from build123d import *

# Parameters (mm, degrees)
SKETCH1_W            = 85.09
SKETCH1_H            = 56.64
BOSS_EXTRUDE1_DEPTH  = 2
SKETCH3_W            = 6
SKETCH3_H            = 2
BOSS_EXTRUDE4_DEPTH  = 6
SKETCH4_R            = 1.27
CUT_EXTRUDE3_DEPTH   = 6
SKETCH5_W            = 6
SKETCH5_H            = 2
BOSS_EXTRUDE5_DEPTH  = 6
SKETCH7_R            = 1.27
CUT_EXTRUDE4_DEPTH   = 6
SKETCH8_W            = 6
SKETCH8_H            = 2
BOSS_EXTRUDE6_DEPTH  = 6
SKETCH9_W            = 6
SKETCH9_H            = 2
BOSS_EXTRUDE7_DEPTH  = 6
SKETCH10_R           = 1.27
CUT_EXTRUDE5_DEPTH   = 6
SKETCH11_R           = 1.27
CUT_EXTRUDE6_DEPTH   = 6
FILLET5_R            = 2
SKETCH12_W           = 33.5
SKETCH12_H           = 5.2
BOSS_EXTRUDE8_DEPTH  = 15
SKETCH14_W           = 33.4
SKETCH14_H           = 5
CUT_EXTRUDE9_DEPTH   = 6
SKETCH15_W           = 5
SKETCH15_H           = 33
BOSS_EXTRUDE9_DEPTH  = 9
SKETCH16_W           = 85
SKETCH16_H           = 55
BOSS_EXTRUDE10_DEPTH = 3.5


with BuildPart() as part:
    # Sketch1 → Boss-Extrude1 (new body)
    with BuildSketch(Plane(origin=(0, 0, 0), x_dir=(1, 0, 0), z_dir=(0, 1, 0))):
        Rectangle(SKETCH1_W, SKETCH1_H)
    extrude(amount=BOSS_EXTRUDE1_DEPTH)

    # Sketch3 → Boss-Extrude4 (add)
    with BuildSketch(Plane(origin=(42.545, 0, 0), x_dir=(0, 0, -1), z_dir=(1, 0, 0))):
        with Locations((-25.32, 1)):
            Rectangle(SKETCH3_W, SKETCH3_H)
    extrude(amount=BOSS_EXTRUDE4_DEPTH)

    # Sketch4 → Cut-Extrude3 (cut)
    with BuildSketch(Plane(origin=(0, 2, 0), x_dir=(1, 0, 0), z_dir=(0, 1, 0))):
        with Locations((45.545, -25.32)):
            Circle(SKETCH4_R)
    extrude(amount=-CUT_EXTRUDE3_DEPTH, mode=Mode.SUBTRACT)

    # Sketch5 → Boss-Extrude5 (add)
    with BuildSketch(Plane(origin=(42.545, 0, 0), x_dir=(0, 0, -1), z_dir=(1, 0, 0))):
        with Locations((25.32, 1)):
            Rectangle(SKETCH5_W, SKETCH5_H)
    extrude(amount=BOSS_EXTRUDE5_DEPTH)

    # Sketch7 → Cut-Extrude4 (cut)
    with BuildSketch(Plane(origin=(0, 2, 0), x_dir=(1, 0, 0), z_dir=(0, 1, 0))):
        with Locations((45.545, 25.32)):
            Circle(SKETCH7_R)
    extrude(amount=-CUT_EXTRUDE4_DEPTH, mode=Mode.SUBTRACT)

    # Sketch8 → Boss-Extrude6 (add)
    with BuildSketch(Plane.ZY.offset(42.545)):
        with Locations((-25.32, 1)):
            Rectangle(SKETCH8_W, SKETCH8_H)
    extrude(amount=BOSS_EXTRUDE6_DEPTH)

    # Sketch9 → Boss-Extrude7 (add)
    with BuildSketch(Plane.ZY.offset(42.545)):
        with Locations((25.32, 1)):
            Rectangle(SKETCH9_W, SKETCH9_H)
    extrude(amount=BOSS_EXTRUDE7_DEPTH)

    # Sketch10 → Cut-Extrude5 (cut)
    with BuildSketch(Plane(origin=(0, 2, 0), x_dir=(1, 0, 0), z_dir=(0, 1, 0))):
        with Locations((-45.545, 25.32)):
            Circle(SKETCH10_R)
    extrude(amount=-CUT_EXTRUDE5_DEPTH, mode=Mode.SUBTRACT)

    # Sketch11 → Cut-Extrude6 (cut)
    with BuildSketch(Plane(origin=(0, 2, 0), x_dir=(1, 0, 0), z_dir=(0, 1, 0))):
        with Locations((-45.545, -25.32)):
            Circle(SKETCH11_R)
    extrude(amount=-CUT_EXTRUDE6_DEPTH, mode=Mode.SUBTRACT)

    # Fillet5
    fillet5_edges = [part.edges().sort_by_distance(p)[0] for p in [
        (48.545, 1, 28.32),
        (48.545, 1, 22.32),
        (48.545, 1, -28.32),
        (48.545, 1, -22.32),
        (-48.545, 1, -28.32),
        (-48.545, 1, -22.32),
        (-48.545, 1, 28.32),
        (-48.545, 1, 22.32),
    ]]
    fillet(fillet5_edges, radius=FILLET5_R)

    # Sketch12 → Boss-Extrude8 (add)
    with BuildSketch(Plane.XZ):
        with Locations((-24.795, -24.72)):
            Rectangle(SKETCH12_W, SKETCH12_H)
    extrude(amount=BOSS_EXTRUDE8_DEPTH)

    # Sketch14 → Cut-Extrude9 (cut)
    with BuildSketch(Plane.XZ.offset(15)):
        with Locations((-24.845, -24.72)):
            Rectangle(SKETCH14_W, SKETCH14_H)
    extrude(amount=-CUT_EXTRUDE9_DEPTH, mode=Mode.SUBTRACT)

    # Sketch15 → Boss-Extrude9 (add)
    with BuildSketch(Plane.XZ):
        with Locations((-37.045, 0.82)):
            Rectangle(SKETCH15_W, SKETCH15_H)
    extrude(amount=BOSS_EXTRUDE9_DEPTH)

    # Sketch16 → Boss-Extrude10 (add)
    with BuildSketch(Plane(origin=(0, 2, 0), x_dir=(1, 0, 0), z_dir=(0, 1, 0))):
        Rectangle(SKETCH16_W, SKETCH16_H)
    extrude(amount=BOSS_EXTRUDE10_DEPTH)


solid = part.part
Input: part model. Units: mm. Frame: model coordinates. A direction names the side the tool comes from. Round coordinates to 2 decimals unless told otherwise and drop trailing zeros. Loops run counter-clockwise (first coordinate to the right, second up) from the corner with the lowest first, then second, coordinate; pieces in that order, holes last. Notation, with made-up numbers: (73, -23) -> (108, -23) arc R27 cw to (108, 3) -> close; hole circle Ø2 at (-24, 34.25). An arc over 180 degrees is marked (long way). Answer as a JSON object with one key per item and string values. Group by question number.
1) Section query D-D on z = -19.5. Output: boundary loops of the cut face in (x, y) (3 decimals).
2) Section query A-A on z = -25.32. Output: boundary loops of the cut face in (x, y) (3 decimals).
3) Section query C-C on y = -4.5. Output: boundary loops of the cut face in (x, z) (3 decimals), plus the area to 3 significant figures.
4) Ray query, L1, parallel to X at y = 1.4, z = 25.32 (3 decimals); L2, parallel to Z at x = -18, y = -4; L3, parallel to Y at x = -1.5, z = 18. Return the intervals inside material, ascending.
5) Reachability of faces 5 (the flat face through (-25, -7, -27.32)), 6 (the flat face through (-25, -9, -25)), 7 (the flat face through (42.545, 1, 0)), 8 (the flat face through (-45, 1, -22.32)), 9 (the cylindrical face through (-46.553, 1.014, 26.093)) from +Z, -Z, +X, -X, +Y, -Y: full face, straight path, thin tool, end or side. Return the list, or none.
6) Pin query (flat end, axial travel): pin 1 (1.5 mm diameter, centred on y = -12, z = -25, fed in from -X) (3 decimals); pin 2 (4 mm diameter, centred on y = 0, z = -0.5, fed in from -X) (3 decimals); pin 3 (1.8 mm diameter, centred on y = 4.5, z = -5.5, fed in from +X); pin 4 (6 mm diameter, centred on x = -18.5, z = -21.5, fed in from -Y). Return the tip coordinate at first contact, or that it passes through.
7) Section query B-B on x = -18. Output: boundary loops of the cut face in (y, z).
8) Draft query along Z for faces 1 (the cylindrical face through (-47.975, 1.014, 27.719)), 2 (the flat face through (-8.045, -7, -25)), 3 (the flat face through (45, 1, -22.32)), 4 (the flat face through (-45, 1, 22.32)). Return one class per face: +Z half, -Z half, draft (parallel to the pull), parting line (faces both ways), or undercut.
Reply:
{
 "1": {"outline": "(-42.545, 0) -> (42.545, 0) -> (42.545, 2) -> (42.5, 2) -> (42.5, 5.5) -> (-42.5, 5.5) -> (-42.5, 2) -> (-42.545, 2) -> close"},
 "2": {"outline": "(-48.545, 0) -> (-46.815, 0) -> (-46.815, 2) -> (-48.545, 2) -> close; (-44.275, 0) -> (-41.545, 0) -> (-41.545, -9) -> (-8.145, -9) -> (-8.145, -15) -> (-8.045, -15) -> (-8.045, 0) -> (44.275, 0) -> (44.275, 2) -> (42.5, 2) -> (42.5, 5.5) -> (-42.5, 5.5) -> (-42.5, 2) -> (-44.275, 2) -> close; (46.815, 0) -> (48.545, 0) -> (48.545, 2) -> (46.815, 2) -> close"},
 "3": {"outline": "(-41.545, -27.32) -> (-8.045, -27.32) -> (-8.045, -22.12) -> (-41.545, -22.12) -> close; (-39.545, -15.68) -> (-34.545, -15.68) -> (-34.545, 17.32) -> (-39.545, 17.32) -> close", "area": "339 mm2"},
 "4": {"L1": "x = -48.545 to -46.815, -44.275 to 44.275, 46.815 to 48.545", "L2": "z = -27.32 to -22.12", "L3": "y = 0 to 5.5"},
 "5": {"face 5": "-Z, +X, -X, -Y", "face 6": "-X, -Y", "face 7": "+X, +Y, -Y", "face 8": "-X, +Y, -Y", "face 9": "+Y, -Y"},
 "6": {"pin 1": "stops at x = -8.145", "pin 2": "stops at x = -42.545", "pin 3": "stops at x = 42.5", "pin 4": "stops at y = -15"},
 "7": {"outline": "(-15, -27.32) -> (0, -27.32) -> (0, -28.32) -> (2, -28.32) -> (2, -27.5) -> (5.5, -27.5) -> (5.5, 27.5) -> (2, 27.5) -> (2, 28.32) -> (0, 28.32) -> (0, -22.12) -> (-15, -22.12) -> (-15, -22.22) -> (-9, -22.22) -> (-9, -27.22) -> (-15, -27.22) -> close"},
 "8": {"face 1": "+Z half", "face 2": "draft", "face 3": "undercut", "face 4": "undercut"}
}
